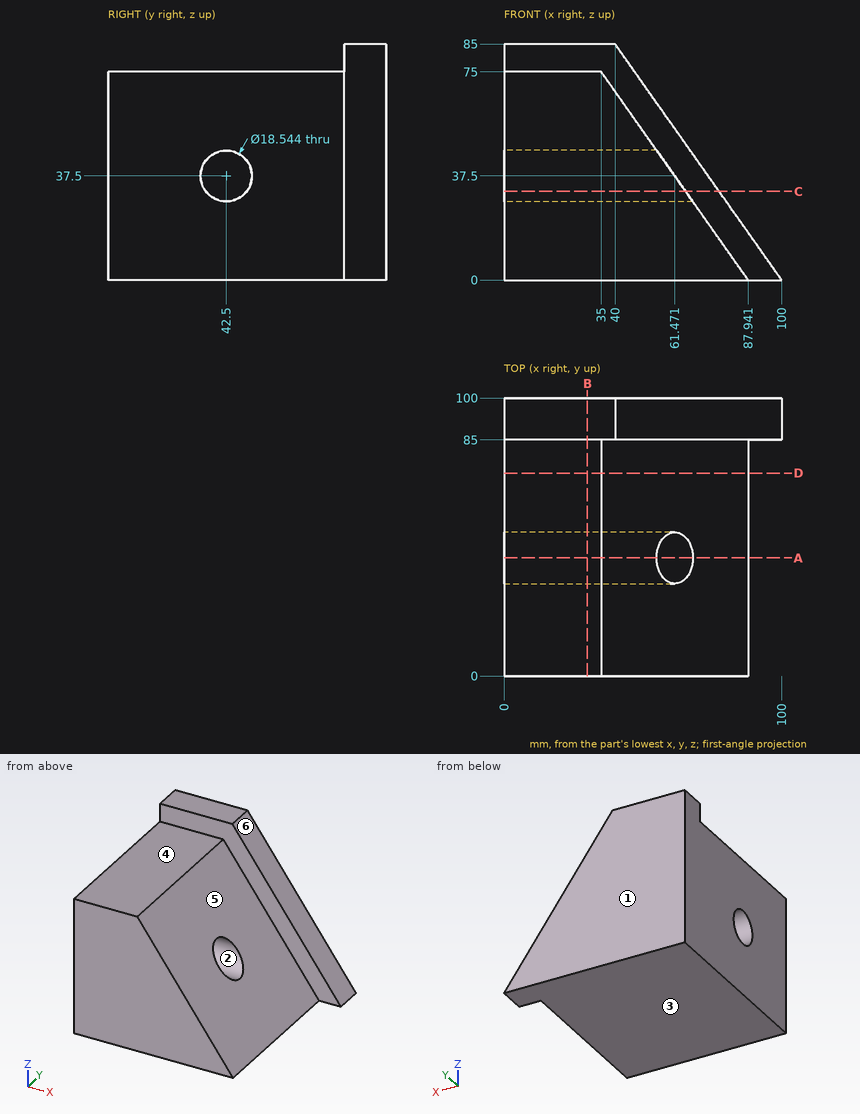
Here's the drawing with two shaded views (mm, measured from the low corner). I have some questions. A direction names the side the tool comes from. Round coordinates to 2 decimals unless told otherwise and drop trailing zeros. Write each loop counter-clockwise with the first axis right and the second up, starting at its lowest first coordinate (ties: lowest second). Pieces come first, ordered by that corner, then holes.
(1) Suppose I cut it at D-D on y = 73. Write out the boundary of the cut face in (x, z).
Findings below:
outline: (0, 0) - (87.94, 0) - (35, 75) - (0, 75) - close
(2) If I drill on probe 1 along Y at (x, z) = (20.5, 37.5); probe 2 along Z at (x, y) = (29.5, 42.5); probe 3 along Z at (x, y) = (15.5, 79.5), over which ranges is the centre line in solid material (lowest first)?
Findings below:
probe 1: y = 0 to 33.23, 51.77 to 100
probe 2: z = 0 to 28.23, 46.77 to 75
probe 3: z = 0 to 75
(3) Suppose I cut it at B-B on x = 30. Write out the boundary of the cut face in (y, z) (1 decimal).
Findings below:
outline: (0, 0) - (100, 0) - (100, 85) - (85, 85) - (85, 75) - (0, 75) - close; hole circle Ø18.5 at (42.5, 37.5)
(4) Which directions (+Z, -Z, +X, -X, +Y, -Y) give clear straight access to the entire face, cutting with the end or side of a thin tool? Please do the marked faces 4, 5 and 6.
Findings below:
face 4: +Z, +X, -X, -Y
face 5: +Z, +X, -Y
face 6: +Z, +X, +Y, -Y
(5) Suppose I cut it at A-A on y = 42.5. Write out the boundary of the cut face in (x, z) (1 decimal).
Findings below:
outline: (0, 0) - (87.9, 0) - (68, 28.2) - (0, 28.2) - close; (0, 46.8) - (54.9, 46.8) - (35, 75) - (0, 75) - close
(6) Thinking about a two-plate mould opening in Y: for the marked faces 1, 2 and 3, which applies, +Y half, -Y half, draft (parallel to the pull), parting line (faces both ways), or undercut?
Findings below:
face 1: +Y half
face 2: undercut
face 3: draft
(7) Suppose I cut it at C-C on z = 32. Write out the boundary of the cut face in (x, y) (1 decimal), and give its area (3 significant figures).
Findings below:
outline: (0, 0) - (65.4, 0) - (65.4, 35) - (0, 35) - close; (0, 50) - (65.4, 50) - (65.4, 85) - (77.4, 85) - (77.4, 100) - (0, 100) - close
area: 5,740 mm2
(8) For pin 1 (2 mm diameter, centred on y = 30, z = 66, fed in from +X); pin 2 (8 mm diameter, centred on y = 32, z = 63.5, fed in from +X); pin 3 (1.5 mm diameter, centred on x = 73.5, y = 35.5, fed in from -Z); pin 4 (8 mm diameter, centred on x = 55.5, y = 48.5, fed in from +Z) (1 decimal), each with a flat end and sliding along its axis, tell me the tip position at first contact or that it passes through.
Findings below:
pin 1: stops at x = 42.06
pin 2: stops at x = 45.94
pin 3: stops at z = 0
pin 4: stops at z = 51.6
